Input: part model. Units: mm. Frame: model coordinates. A direction names the side the tool comes from. Give positions to 0.01 mm unless a question says otherwise; leave off trailing zeros. Order: outer loops, then holes, each group sorted by start corner. A loop starts at its lowest first (then second) coordinate and runs counter-clockwise, first axis right, second up. Notation, with made-up numbers: (74.5, 68.5) - (120.5, 68.5) arc R28 cw to (120.5, 92.5) - close; hole circle Ø8 at (83, -30.5). An arc over 180 degrees is marked (long way). Answer in a Markdown table with one row per item. Add a question column.
1. Mould query, pull axis X, two halves, no side actions, for faces 4 (the face through (-57.208, 50.014, -0.342)), 5 (the face through (-65, 51, 0)), 6 (the face through (-74.719, 41, 0)), 7 (the face through (-67.788, 40, 0)). Classes: released by +X, released by -X, zero draft, split by the parting line, or undercut.
2. Section query A-A on z = 0.75. Return loops of the section in (x, y), and give its area (3 significant figures).
3. Contact query for flat-ended pins moving along their axis: pin 1 (3 mm diameter, centred on x = -68, z = 3.5, fed in from -Y); pin 2 (6 mm diameter, centred on x = -59, z = 0.5, fed in from -Y); pin 3 (1.5 mm diameter, centred on x = -61, z = -3.5, fed in from -Y). Output: stop coordinate, or through.
4. Access query for faces 1 (the face through (-57, 47, 4.25)), 2 (the face through (-64, 44, 0)), 3 (the face through (-67, 45, -5.25)). Directions: +Z, -Z, +X, -X, +Y, -Y. A direction counts if a zero-diameter tool reaches every point of the face in a straight line with its end or side. Return the directions, or none.
5. Section query D-D on z = 3.5. Return loops of the section in (x, y).
6. Section query B-B on x = -61.75. Return loops of the section in (y, z).
7. Section query C-C on y = 40. Return loops of the section in (x, z), and give its area (3 significant figures).
8. Ray query, line 1 (Z direction, x = -58.75, y = 46.75); line 2 (Y direction, x = -65.25, z = 3); line 3 (X direction, y = 41.5, z = 0.25). Return the intervals inside material, ascending. Write a range as [from, to].
```python
from build123d import *

# Parameters (mm, degrees)
EXTRUSION1_DEPTH        = 5.25
EXTRUSION2_DEPTH        = 5
ESQUISSE3_R             = 2
ENL_V_MAT_EXTRU_1_DEPTH = 2
CHANFREIN1_SIZE         = 2


with BuildPart() as part:
    # Esquisse1 → Extrusion1 (new, symmetric)
    with BuildSketch(Plane.XY):
        Polygon((-55.719296469, 49), (-67.787598819, 49), (-67.787598819, 35.452607164), (-71.187598819, 35.452607164), (-71.187598819, 30.452607164), (-74.719296469, 30.452607164), (-74.719296469, 51), (-55.719296469, 51), align=None)
    extrude(amount=EXTRUSION1_DEPTH, both=True)

    # Esquisse2 → Extrusion2 (add)
    with BuildSketch(Plane.XZ.offset(-49)):
        with BuildLine():
            Line((-55.719296469, 5.25), (-69.802319992, 5.25))
            Line((-69.802319992, 5.25), (-69.802319992, -5.25))
            Line((-69.802319992, -5.25), (-55.719296469, -5.25))
            Line((-55.719296469, -5.25), (-55.719296469, -4.25))
            Line((-55.719296469, -4.25), (-59.219296469, -4.25))
            ThreePointArc((-59.219296469, -4.25), (-63.469296469, 0), (-59.219296469, 4.25))
            Line((-59.219296469, 4.25), (-55.719296469, 4.25))
            Line((-55.719296469, 4.25), (-55.719296469, 5.25))
        make_face()
    extrude(amount=EXTRUSION2_DEPTH)

    # Esquisse3 → Enlèv. mat.-Extru.1 (cut)
    with BuildSketch(Plane(origin=(0, 51, 0), x_dir=(-1, 0, 0), z_dir=(0, 1, 0))):
        with Locations(Location((59.190865046, -0.081564641, 0), (0, 0, 90))):
            Circle(ESQUISSE3_R)
    extrude(amount=-ENL_V_MAT_EXTRU_1_DEPTH, mode=Mode.SUBTRACT)

    # Chanfrein1
    chanfrein1_edges = [part.edges().sort_by_distance(p)[0] for p in [
        (-55.719296469, 44, -4.75),
        (-55.719296469, 44, 4.75),
    ]]
    chamfer(chanfrein1_edges, length=CHANFREIN1_SIZE)


solid = part.part
```
Answer:
| question | item | result |
|---|---|---|
| 1 | face 4 | undercut |
| 1 | face 5 | zero draft |
| 1 | face 6 | released by -X |
| 1 | face 7 | released by +X |
| 2 | outline | (-74.72, 30.45) - (-71.19, 30.45) - (-71.19, 35.45) - (-67.79, 35.45) - (-67.79, 44) - (-63.4, 44) - (-63.4, 49) - (-61.01, 49) - (-61.01, 51) - (-74.72, 51) - close; (-57.37, 49) - (-55.72, 49) - (-55.72, 51) - (-57.37, 51) - close |
| 2 | area | 164 mm² |
| 3 | pin 1 | stops at y = 35.45 |
| 3 | pin 2 | stops at y = 49 |
| 3 | pin 3 | stops at y = 44 |
| 4 | face 1 | +X, -Y |
| 4 | face 2 | +Z, -Z, +X, -Y |
| 4 | face 3 | -Z, +X, -X, +Y, -Y |
| 5 | outline | (-74.72, 30.45) - (-71.19, 30.45) - (-71.19, 35.45) - (-67.79, 35.45) - (-67.79, 44) - (-61.63, 44) - (-61.63, 49) - (-55.72, 49) - (-55.72, 51) - (-74.72, 51) - close |
| 6 | outline | (44, -5.25) - (51, -5.25) - (51, 5.25) - (44, 5.25) - (44, 3.41) - (49, 3.41) - (49, -3.41) - (44, -3.41) - close |
| 7 | outline | (-74.72, -5.25) - (-67.79, -5.25) - (-67.79, 5.25) - (-74.72, 5.25) - close |
| 7 | area | 72.8 mm² |
| 8 | line 1 | z = [-5.25, -4.25], [4.25, 5.25] |
| 8 | line 2 | y = [44, 51] |
| 8 | line 3 | x = [-74.72, -67.79] |
